Geometry: final body of the model. Coordinates: model frame, mm. Give positions to 0.01 mm unless a question says otherwise; leave off trailing zeros. Write each loop counter-clockwise with the first axis right and the second up, starting at its lowest first coordinate (ties: lowest second). Pieces come first, ordered by that corner, then holes.
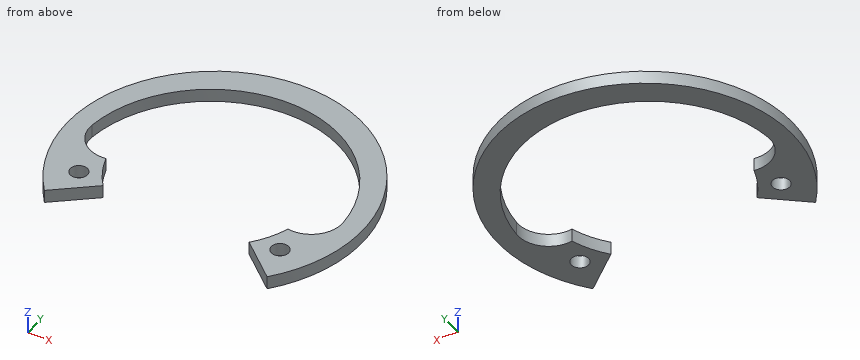
```python
from build123d import *

# Parameters (mm, degrees)
SKETCH1_R           = 1
BOSS_EXTRUDE1_DEPTH = 1.5


with BuildPart() as part:
    # Sketch1 → Boss-Extrude1 (new body)
    with BuildSketch(Plane.XY):
        with BuildLine():
            Line((-13.022755533, -10.927389365), (-8.541395541, -7.167081848))
            ThreePointArc((-8.541395541, -7.167081848), (-9.783859128, -5.347765941), (-10.644354895, -3.319669993))
            ThreePointArc((-10.644354895, -3.319669993), (-13.596382147, -2.37892663), (-14.690850544, 0.51962506))
            ThreePointArc((-14.690850544, 0.51962506), (0, 13.95), (14.690850544, 0.51962506))
            ThreePointArc((14.690850544, 0.51962506), (13.596382147, -2.37892663), (10.644354895, -3.319669993))
            ThreePointArc((10.644354895, -3.319669993), (9.783859128, -5.347765941), (8.541395541, -7.167081848))
            Line((8.541395541, -7.167081848), (13.022755533, -10.927389365))
            ThreePointArc((13.022755533, -10.927389365), (0, 17), (-13.022755533, -10.927389365))
        make_face()
        with Locations((-11.762324169, -6.547389365)):
            Circle(SKETCH1_R, mode=Mode.SUBTRACT)
        with Locations(Location((11.762324169, -6.547389365, 0), (0, 0, 180))):
            Circle(SKETCH1_R, mode=Mode.SUBTRACT)
    extrude(amount=BOSS_EXTRUDE1_DEPTH)


solid = part.part
```
Item 1: Section A-A, the plane y = 10.25. Return the cut outline in (x, z).
Found:
outline: (-13.56, 0) - (-9.77, 0) - (-9.77, 1.5) - (-13.56, 1.5) - close; (9.77, 0) - (13.56, 0) - (13.56, 1.5) - (9.77, 1.5) - close
Item 2: Section D-D, the plane y = 0. Return the cut outline in (x, z).
Found:
outline: (-17, 0) - (-14.7, 0) - (-14.7, 1.5) - (-17, 1.5) - close; (14.7, 0) - (17, 0) - (17, 1.5) - (14.7, 1.5) - close
Item 3: Line query: L1, parallel to X at y = 0.5, z = 0.9; L2, parallel to Y at x = 11.5, z = 1.4; L3, parallel to Y at x = 0, z = 0.55. Output: solid intervals per line, ascending.
Found:
L1: x = -16.99 to -14.69, 14.69 to 16.99
L2: y = -9.65 to -7.51, -5.58 to -3.34, 8.44 to 12.52
L3: y = 13.95 to 17
Item 4: Pin query (flat end, axial travel): pin 1 Ø2.5 at (x, y) = (-11.76, -6.55) entering from +Z. Return the tip coordinate at first contact, or that it passes through.
Found:
pin 1: stops at z = 1.5
Item 5: Section B-B, the plane z = 0.35. Return the cut outline in (x, y), plus the area to 3 significant figures.
Found:
outline: (-14.69, 0.52) arc R14.75 cw to (14.69, 0.52) arc R3.56 cw to (10.64, -3.32) arc R11.15 cw to (8.54, -7.17) - (13.02, -10.93) arc R17 ccw (long way) to (-13.02, -10.93) - (-8.54, -7.17) arc R11.15 cw to (-10.64, -3.32) arc R3.56 cw to start; hole circle Ø2 at (-11.76, -6.55); hole circle Ø2 at (11.76, -6.55)
area: 225 mm2
Item 6: Section C-C, the plane x = 0. Return the cut outline in (y, z), plus the area to 4 significant figures.
Found:
outline: (13.95, 0) - (17, 0) - (17, 1.5) - (13.95, 1.5) - close
area: 4.575 mm2
